Answer from the drawing. Dimensions are ordinates in mm from the lowest x, y and z of the part. A direction names the side the tool comes from. Coordinates: 2 decimals unless noted, no trailing zeros. Write each loop counter-clockwise with the first axis right and the second up, starting at its lowest first coordinate (ties: lowest second). Pieces come first, ordered by that corner, then holes. Notation, with made-up numbers: (13.5, 13.25) -> (61.5, 13.25) arc R10 cw to (61.5, 19.25) -> close; hole circle Ø9 at (-0.5, 61.25). An arc over 180 degrees is marked (long way). One line per item, written item: value. Start each with the question number.
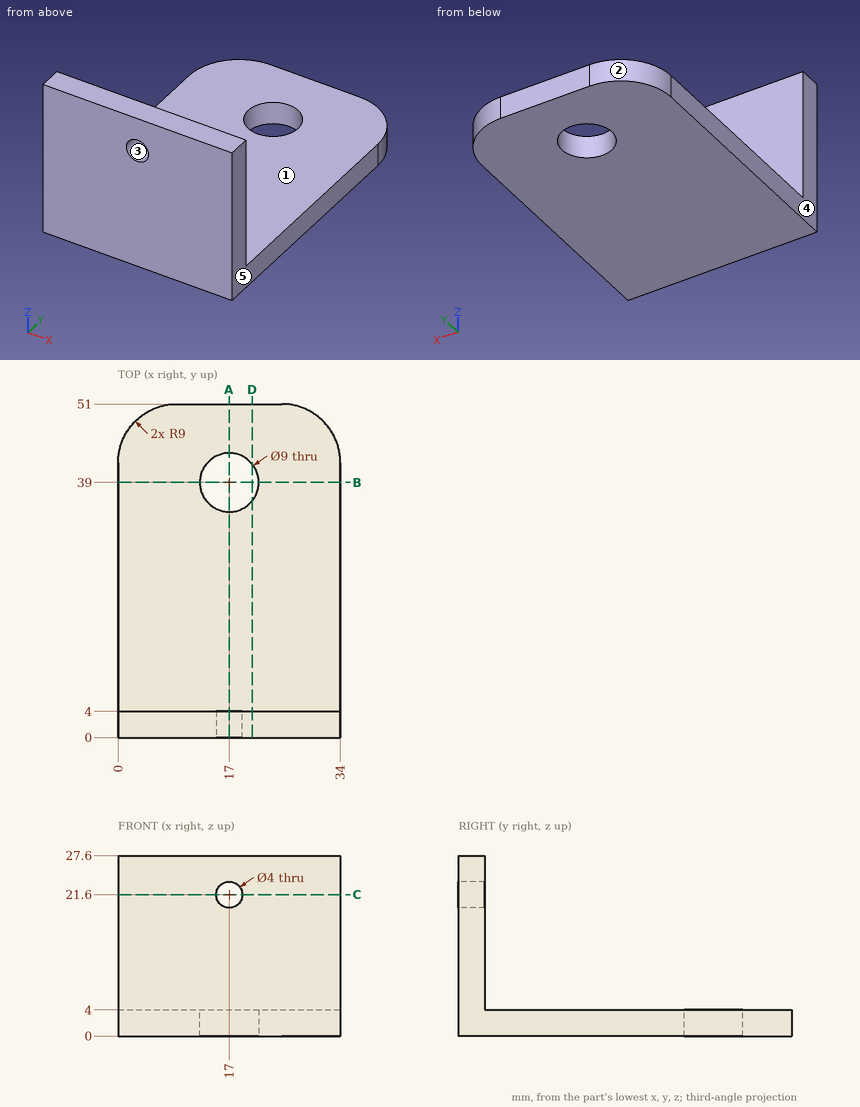
1. A cutting plane is placed at A-A on x = 17. Give the vertices of the cut face in (y, z), then the cut area to 3 significant figures.
2. A tool of negligible diameter and unlimited length cuts with its end or side. For the marked faces 1 and 2, from which of +Z, -Z, +X, -X, +Y, -Y can it reach the whole face along a straight path? Write none if from no direction.
3. A cutting plane is placed at C-C on z = 21.6. Give the vertices of the cut face in (x, y), then the cut area to 3 significant figures.
4. A cutting plane is placed at B-B on y = 39. Give the vertices of the cut face in (x, z).
5. A cutting plane is placed at D-D on x = 20.5. Give the vertices of the cut face in (y, z).
6. Given pin 1 (1.5 mm diameter, centred on x = 25.5, y = 31.5, fed in from +Z); pin 2 (8 mm diameter, centred on x = 17, y = 39, fed in from -Z); pin 3 (12 mm diameter, centred on x = 10.5, z = 16.5, fed in from +Y), each flat-ended and moving along its own axis, determine where each tip first touches the part or whether it passes through.
7. For a pull along X with two mould halves and no side action, classify the marked faces 3, 4 and 5 as +X half, -X half, draft (parallel to the pull), parting line (faces both ways), or undercut.
8. Find the intervals of material crossed by probe 1 along Y at (x, z) = (17, 2.95); probe 2 along X at (y, z) = (2.35, 21.6); probe 3 along Z at (x, y) = (17, 2), in increasing order. Write a range as from..to.
Derived:
1. outline: (0, 0) -> (34.5, 0) -> (34.5, 4) -> (4, 4) -> (4, 19.6) -> (0, 19.6) -> close; (0, 23.6) -> (4, 23.6) -> (4, 27.6) -> (0, 27.6) -> close; (43.5, 0) -> (51, 0) -> (51, 4) -> (43.5, 4) -> close
1. area: 246 mm2
2. face 1: +Z, +X, -X, +Y
2. face 2: +Z, -Z, -X, +Y
3. outline: (0, 0) -> (15, 0) -> (15, 4) -> (0, 4) -> close; (19, 0) -> (34, 0) -> (34, 4) -> (19, 4) -> close
3. area: 120 mm2
4. outline: (0, 0) -> (12.5, 0) -> (12.5, 4) -> (0, 4) -> close; (21.5, 0) -> (34, 0) -> (34, 4) -> (21.5, 4) -> close
5. outline: (0, 0) -> (36.17, 0) -> (36.17, 4) -> (4, 4) -> (4, 27.6) -> (0, 27.6) -> close; (41.83, 0) -> (51, 0) -> (51, 4) -> (41.83, 4) -> close
6. pin 1: stops at z = 4
6. pin 2: passes through
6. pin 3: stops at y = 4
7. face 3: undercut
7. face 4: -X half
7. face 5: +X half
8. probe 1: y = 0..34.5, 43.5..51
8. probe 2: x = 0..15, 19..34
8. probe 3: z = 0..19.6, 23.6..27.6
